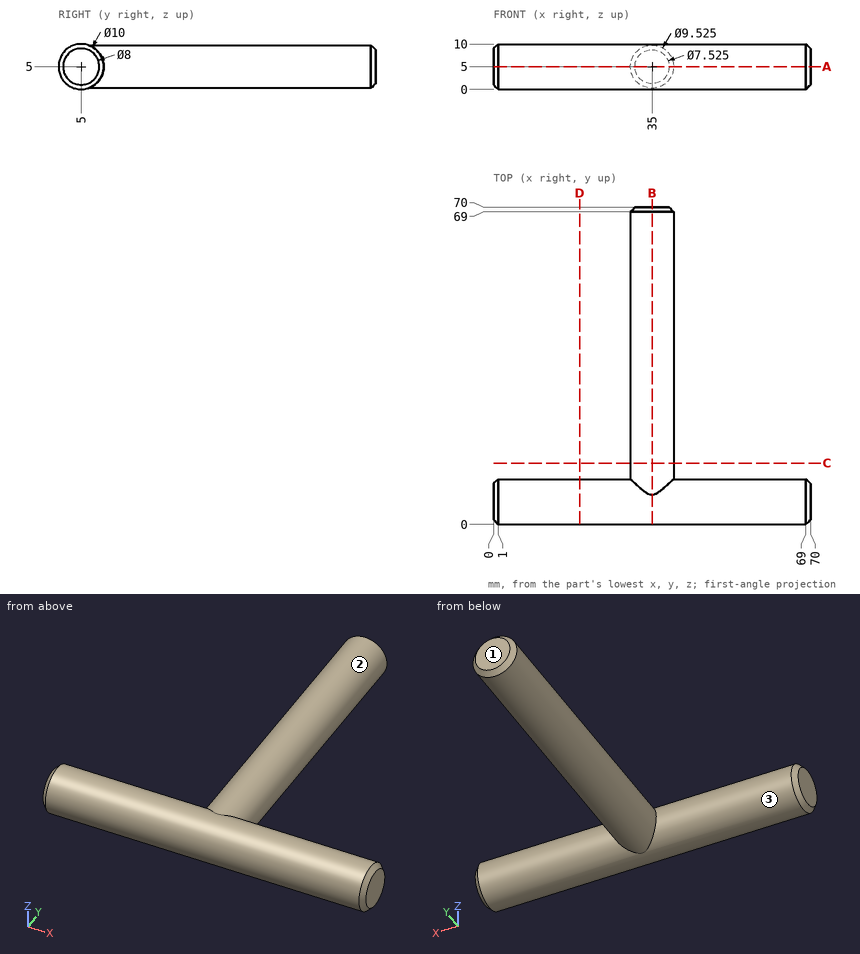
Job drawing, mm, ordinate dimensions from the low corner. One solid piece. A direction names the side the tool comes from. Round coordinates to 2 decimals unless told otherwise and drop trailing zeros. Loops run counter-clockwise (first coordinate to the right, second up) from the corner with the lowest first, then second, coordinate; pieces in that order, holes last. Notation, with made-up numbers: (33, 60.25) -> (47, 60.25) arc R11 ccw to (47, 73.25) -> close; hole circle Ø8 at (-8.5, -9.5). An arc over 180 degrees is marked (long way). Use a Markdown table: item, result.
1) Drop flat-ended pins along their axis: pin 1 Ø5 at (y, z) = (56.5, 2.5) entering from -X; pin 2 Ø1.5 at (y, z) = (14, 3) entering from -X; pin 3 Ø1.5 at (x, z) = (63, 2.5) entering from -Y. Give the stop position or say it passes through.
The answers:
| item | result |
|---|---|
| pin 1 | stops at x = 30.24 |
| pin 2 | stops at x = 30.4 |
| pin 3 | stops at y = 0.32 |
2) Cut at C-C, the plane y = 13.5. List the corners of the cut face in (x, z) (1 decimal), and give its area (3 significant figures).
The answers:
| item | result |
|---|---|
| outline | circle Ø9.5 at (35, 5) |
| area | 71.3 mm2 |
3) Cut at D-D, the plane x = 19. List the corners of the cut face in (y, z), and give its area (3 significant figures).
The answers:
| item | result |
|---|---|
| outline | circle Ø10 at (5, 5) |
| area | 78.5 mm2 |
4) Cut at A-A, the plane z = 5. List the corners of the cut face in (x, y), and give its area (3 significant figures).
The answers:
| item | result |
|---|---|
| outline | (0, 1) -> (1, 0) -> (69, 0) -> (70, 1) -> (70, 9) -> (69, 10) -> (39.76, 10) -> (39.76, 69) -> (38.76, 70) -> (31.24, 70) -> (30.24, 69) -> (30.24, 10) -> (1, 10) -> (0, 9) -> close |
| area | 1,270 mm2 |
5) Tool access for the marked faces 1, 2 and 3: list every direction of +Z, -Z, +X, -X, +Y, -Y with a clear straight run to the whole face (end or side of a thin tool).
The answers:
| item | result |
|---|---|
| face 1 | +Z, -Z, +X, -X, +Y |
| face 2 | +Y |
| face 3 | none |
6) Cut at B-B, the plane x = 35. List the corners of the cut face in (y, z).
The answers:
| item | result |
|---|---|
| outline | (6.52, 0.24) -> (69, 0.24) -> (70, 1.24) -> (70, 8.76) -> (69, 9.76) -> (6.52, 9.76) arc R5 ccw (long way) to start |
7) Probe line 1 (X direction, y = 12, z = 5.25); line 2 (Y direction, x = 56, z = 4.75); line 3 (Z direction, x = 33, y = 49.5). List the from-to ranges inside material, lowest first. Write a range as [from, to].
The answers:
| item | result |
|---|---|
| line 1 | x = [30.24, 39.76] |
| line 2 | y = [0.01, 9.99] |
| line 3 | z = [0.68, 9.32] |
